Can you work these out from the model? Positions are in its coordinate system, mm. Coordinates: 2 decimals unless noted, no trailing zeros. Order: outer loops, then holes, each group sorted by start corner. A loop starts at its lowest first (then second) coordinate and runs counter-clockwise, first axis right, second up. Notation, with made-up numbers: M -3.75,10.5 L 12.25,10.5 A13 ccw 12.25,16.5 Z; hole C 51,72 d1. An arc over 180 degrees is marked long. Answer as CSV lines item,"result". Start each with the question number.
1. If we section it at B-B (z = 2.25): List the corners of the cut face in (x, y) for me (3 decimals), plus the area to 3 significant figures.
2. If we section it at A-A (x = 0.25): List the corners of the cut face in (y, z) for me (3 decimals).
3. I need wall thicknesses on line 1 along Y through (x, z) = (10.5, 1.5) (3 decimals); line 2 along Y through (x, z) = (-7.25, -0.75) (3 decimals). Which ranges of each line are inside material? Lowest first, please. Write a range as from..to.
4. If we section it at C-C (z = -2): List the corners of the cut face in (x, y) for me (3 decimals), plus the area to 3 significant figures.
```python
from build123d import *

# Parameters (mm, degrees)
F0_W        = 25.4
F0_H        = 6.35
F1_DEPTH    = 101.6
F2_T1_DEPTH = 51.5282991577


# Not quite as in the source:
# - a fillet or chamfer that OpenCascade refuses, or shapes differently, is made with other operations: its cross-section is extruded or revolved along the edge and cut away or added


with BuildPart() as f1:
    # F0 (on Front) → F1 (new body)
    with BuildSketch(Plane.XZ):
        Rectangle(F0_W, F0_H)
    extrude(amount=F1_DEPTH)

    # F2: chamfer of 5.08 on 2 edges, made by hand

    # F2_s2 → F2_t1 (cut)
    with BuildSketch(Plane.YZ.offset(-25.7641495789)):
        Polygon((-96.52, 3.175), (-101.6, -1.905), (-101.6, 3.175), align=None)
        Polygon((-96.52, -3.175), (-101.6, 1.905), (-101.6, -3.175), align=None)
    extrude(amount=F2_T1_DEPTH, mode=Mode.SUBTRACT)


solid = f1.part
```
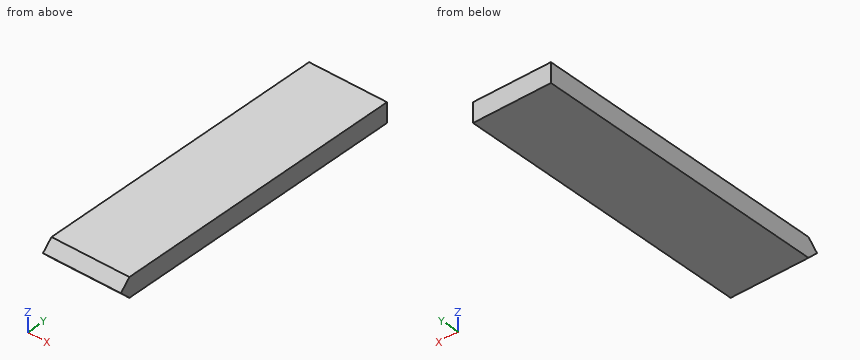
Solved:
1,outline,"M -12.7,-97.445 L 12.7,-97.445 L 12.7,0 L -12.7,0 Z"
1,area,"2,480 mm²"
2,outline,"M -99.695,0 L -96.52,-3.175 L 0,-3.175 L 0,3.175 L -96.52,3.175 Z"
3,line 1,"-98.195..0"
3,line 2,"-98.945..0"
4,outline,"M -12.7,-97.695 L 12.7,-97.695 L 12.7,0 L -12.7,0 Z"
4,area,"2,480 mm²"
